```python
from build123d import *

# Parameters (mm, degrees)
F1_DEPTH = 50.8
F2_R     = 6.217599599
F3_DEPTH = 88.2316216
F4_R     = 2.54


# Not quite as in the source:
# - an extrude ends at something that could not be found from the text; its depth is read off the source's solid


with BuildPart() as f1:
    # F0 (on Front) → F1 (new body)
    with BuildSketch(Plane.XZ):
        with BuildLine():
            Line((1.2967513424, -23.9979514112), (0, 0))
            Line((0, 0), (-63.9691352844, 0))
            Line((-63.9691352844, 0), (-61.5289509296, -30.7046994567))
            Line((-61.5289509296, -30.7046994567), (-6.8309613811, -30.7046994567))
            ThreePointArc((-6.8309613811, -30.7046994567), (-4.3476416049, -25.4359191552), (1.2967513424, -23.9979514112))
        make_face()
    extrude(amount=F1_DEPTH)

    # F2 (on face) → F3 (join, through all)
    with BuildSketch(Plane.XZ.offset(50.8)):
        with Locations((-36.0038354993, -14.3174901605)):
            Circle(F2_R)
    extrude(amount=F3_DEPTH)

    # F4
    f4_edges = [f1.edges().sort_by_distance(p)[0] for p in [
        (-42.221435, -139.031622, -14.31749),
        (-61.528951, -25.4, -30.704699),
        (-63.969135, -25.4, 0),
        (1.296751, -25.4, -23.997951),
        (-6.830961, -25.4, -30.704699),
        (0, -25.4, 0),
        (-31.984568, 0, 0),
        (-62.749043, 0, -15.35235),
        (-34.179956, 0, -30.704699),
        (-4.347642, 0, -25.435919),
        (0.648376, 0, -11.998976),
        (-31.984568, -50.8, 0),
        (0.648376, -50.8, -11.998976),
        (-4.347642, -50.8, -25.435919),
        (-34.179956, -50.8, -30.704699),
        (-62.749043, -50.8, -15.35235),
        (-42.221435, -50.8, -14.31749),
    ]]
    fillet(f4_edges, radius=F4_R)


solid = f1.part
```
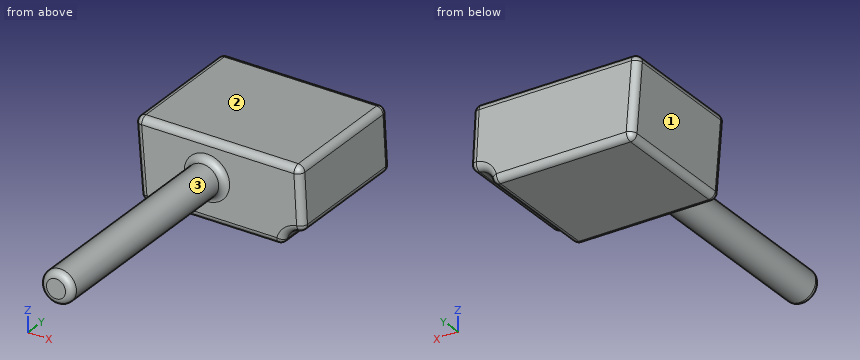
The listing builds one solid part. Answer for the finished solid, in the listing's coordinates (mm). Face numbers are marked on the shaded views. Give positions to 0.01 mm unless a question says otherwise; leave off trailing zeros. Order: outer loops, then holes, each group sorted by start corner. A loop starts at its lowest first (then second) coordinate and runs counter-clockwise, first axis right, second up. Notation, with made-up numbers: (1, 68) - (40, 68) arc R18 ccw to (40, 97) - close; hole circle Ø1 at (2.5, -16). An arc over 180 degrees is marked (long way). Answer in a Markdown table with one row per item. Add a question column.
Q1. Given P1, Ø1, axis at y = -46, z = -26, coming from the -X side; P2, Ø4, axis at x = -40, z = -10, coming from the -Y side; P3, Ø8, axis at y = -110, z = -10, coming from the +X side, each flat-ended and moving along its own axis, determine where each tip first touches the part or whether it passes through.
Q2. The part is cut by section C-C (y = -79.5). Determine the outline of the cut face in (x, z).
Q3. For a pull along X with two mould halves and no side action, classify the marked faces 1, 2 and 3 as released by +X, released by -X, zero draft, split by the parting line, or undercut.
Q4. Find the intervals of material crossed by line 1 along Y through (x, z) = (-26.5, -11); line 2 along X through (y, z) = (-76, -17.5); line 3 along X through (y, z) = (-39, -15), in increasing order. Write a range as [from, to].
Q5. The part is cut by section B-B (y = -12.5). Determine the outline of the cut face in (x, z), then the cut area to 3 significant figures.
Q6. The part is cut by section A-A (x = -57). Determine the outline of the cut face in (y, z), then the cut area to 3 significant figures.
Determined:
| question | item | result |
|---|---|---|
| 1 | P1 | stops at x = -61.94 |
| 1 | P2 | stops at y = -139.02 |
| 1 | P3 | stops at x = -29.79 |
| 2 | outline | circle Ø12.44 at (-36, -14.32) |
| 3 | face 1 | released by -X |
| 3 | face 2 | zero draft |
| 3 | face 3 | split by the parting line |
| 4 | line 1 | y = [-50.8, 0] |
| 4 | line 2 | x = [-41.35, -30.66] |
| 4 | line 3 | x = [-62.78, 0.81] |
| 5 | outline | (-63.75, -2.74) - (-61.71, -28.37) arc R2.54 ccw to (-59.18, -30.7) - (-9.02, -30.7) arc R2.54 ccw to (-6.58, -28.85) arc R6.83 cw to (-1.01, -23.95) arc R2.54 ccw to (1.15, -21.3) - (0.13, -2.4) arc R2.54 ccw to (-2.41, 0) - (-61.22, 0) arc R2.54 ccw to start |
| 5 | area | 1,900 mm² |
| 6 | outline | (-50.8, -28.16) arc R2.54 ccw to (-48.26, -30.7) - (-2.54, -30.7) arc R2.54 ccw to (0, -28.16) - (0, -2.54) arc R2.54 ccw to (-2.54, 0) - (-48.26, 0) arc R2.54 ccw to (-50.8, -2.54) - close |
| 6 | area | 1,550 mm² |
